Read the model definition and answer for the solid it produces. Units are mm, in the model's axes. A direction names the side the tool comes from. Give positions to 0.01 mm unless a question says otherwise; leave off trailing zeros. Loops run counter-clockwise (first coordinate to the right, second up) from the corner with the lowest first, then second, coordinate; pieces in that order, holes last. Notation, with made-up numbers: (-5.75, -28.75) - (4.25, -28.75) arc R23 ccw to (4.25, -1.75) - close; hole circle Ø5 at (81, -27). An arc over 180 degrees is marked (long way). Use a Markdown table: item, result. Add a question column.
Item 1: A cutting plane is placed at B-B (y = 211.5). Give the number of separate pieces and of enclosed holes in the cut face, plus the area to 3 significant figures.
Item 2: Each of these flat-tipped pins is pushed along its axis until it touches: P1, Ø12, axis at x = 0, y = 342.5, coming from the -Z side; P2, Ø2.5, axis at x = 0, y = 119.5, coming from the +Z side; P3, Ø2.5, axis at x = -0.5, y = 263.5, coming from the -Z side. Where does it stop, or does it pass through?
Item 3: A cutting plane is placed at A-A (x = -0.25). Determine the outline of the cut face in (y, z), plus the area to 3 significant figures.
Item 4: For a pull along X with two mould halves and no side action, classify faces 1 (the face through (-3.5, 203, 0)), 2 (the face through (-5, 203, 0)), 3 (the face through (15, 197, -11)), 4 (the face through (0, 203, 5)) as +X half, -X half, draft (parallel to the pull), parting line (faces both ways), or undercut.
Item 5: Which of the six approach directions +Z, -Z, +X, -X, +Y, -Y give full straight-line access (tool end or side, diameter ignored) to faces 5 (the face through (5, 203, 0)), 6 (the face through (0, 203, 3.5)), 7 (the face through (0, 203, -5)), 8 (the face through (-0.1, 400, -4.5)), 9 (the face through (15, 197, 11))?
Item 6: Consider probe 1 along Z at (x, y) = (11.75, 310.5); probe 2 along X at (y, z) = (219, 1.25); probe 3 along X at (y, z) = (240, 7.5). Determine where each line is inside the solid, lowest interval first. Write a range as [from, to].
from build123d import *

# Parameters (mm, degrees)
SKETCH_1_W          = 30
SKETCH_1_H          = 30
EXTRUDE_1_DEPTH     = 400
CUT_EXTRUDE_1_DEPTH = 400
SKETCH_3_W          = 7
SKETCH_3_H          = 7
SKETCH_3_W_2        = 2.5
SKETCH_3_H_2        = 2.5
CUT_EXTRUDE_2_DEPTH = 400


with BuildPart() as part:
    # 草图1 → 凸台-拉伸1 (new body)
    with BuildSketch(Plane(origin=(0, 0, 0), x_dir=(1, 0, 0), z_dir=(0, 1, 0))):
        Rectangle(SKETCH_1_W, SKETCH_1_H)
    extrude(amount=EXTRUDE_1_DEPTH)

    # 草图2 → 切除-拉伸1 (cut)
    with BuildSketch(Plane(origin=(0, 400, 0), x_dir=(1, 0, 0), z_dir=(0, 1, 0))):
        Polygon((-4.004617846, 5), (4.004617846, 5), (9.97363434, 10.969016494), (9.97363434, 13.177944766), (6.476155555, 13.177944766), (5.84989743, 12.551686641), (5.001284858, 13.400299213), (6.600985645, 15), (-6.600985645, 15), (-5.001284858, 13.400299213), (-5.84989743, 12.551686641), (-6.476155555, 13.177944766), (-9.97363434, 13.177944766), (-9.97363434, 10.969016494), align=None)
        Polygon((10.969016494, 9.97363434), (5, 4.004617846), (5, -4.004617846), (10.969016494, -9.97363434), (13.177944766, -9.97363434), (13.177944766, -6.476155555), (12.551686641, -5.84989743), (13.400299213, -5.001284858), (15, -6.600985645), (15, 6.600985645), (13.400299213, 5.001284858), (12.551686641, 5.84989743), (13.177944766, 6.476155555), (13.177944766, 9.97363434), align=None)
        Polygon((-5, -4.004617846), (-5, 4.004617846), (-10.969016494, 9.97363434), (-13.177944766, 9.97363434), (-13.177944766, 6.476155555), (-12.551686641, 5.84989743), (-13.400299213, 5.001284858), (-15, 6.600985645), (-15, -6.600985645), (-13.400299213, -5.001284858), (-12.551686641, -5.84989743), (-13.177944766, -6.476155555), (-13.177944766, -9.97363434), (-10.969016494, -9.97363434), align=None)
        Polygon((9.97363434, -10.969016494), (4.004617846, -5), (-4.004617846, -5), (-9.97363434, -10.969016494), (-9.97363434, -13.177944766), (-6.476155555, -13.177944766), (-5.84989743, -12.551686641), (-5.001284858, -13.400299213), (-6.600985645, -15), (6.600985645, -15), (5.001284858, -13.400299213), (5.84989743, -12.551686641), (6.476155555, -13.177944766), (9.97363434, -13.177944766), align=None)
    extrude(amount=-CUT_EXTRUDE_1_DEPTH, mode=Mode.SUBTRACT)

    # 草图3 → 切除-拉伸2 (cut)
    with BuildSketch(Plane(origin=(0, 400, 0), x_dir=(1, 0, 0), z_dir=(0, 1, 0))):
        Rectangle(SKETCH_3_W, SKETCH_3_H)
        with Locations((12.48681717, -12.48681717)):
            Rectangle(SKETCH_3_W_2, SKETCH_3_H_2)
        with Locations((12.48681717, 12.48681717)):
            Rectangle(SKETCH_3_W_2, SKETCH_3_H_2)
        with Locations((-12.48681717, -12.48681717)):
            Rectangle(SKETCH_3_W_2, SKETCH_3_H_2)
        with Locations((-12.48681717, 12.48681717)):
            Rectangle(SKETCH_3_W_2, SKETCH_3_H_2)
    extrude(amount=-CUT_EXTRUDE_2_DEPTH, mode=Mode.SUBTRACT)


solid = part.part
Geometry says:
| question | item | result |
|---|---|---|
| 1 | separate pieces | 1 |
| 1 | enclosed holes | 5 |
| 1 | area | 236 mm² |
| 2 | P1 | z = -14.4 |
| 2 | P2 | z = 5 |
| 2 | P3 | z = -5 |
| 3 | outline | (0, -5) - (400, -5) - (400, -3.5) - (0, -3.5) - close; (0, 3.5) - (400, 3.5) - (400, 5) - (0, 5) - close |
| 3 | area | 1,200 mm² |
| 4 | face 1 | undercut |
| 4 | face 2 | -X half |
| 4 | face 3 | +X half |
| 4 | face 4 | undercut |
| 5 | face 5 | +X, +Y, -Y |
| 5 | face 6 | +Y, -Y |
| 5 | face 7 | -Z, +Y, -Y |
| 5 | face 8 | +Z, -Z, +X, -X, +Y |
| 5 | face 9 | +Z, -Z, +X, +Y, -Y |
| 6 | probe 1 | [-15, -13.74], [-11.24, -9.97], [9.97, 11.24], [13.74, 15] |
| 6 | probe 2 | [-5, -3.5], [3.5, 5] |
| 6 | probe 3 | [-15, -13.18], [-8.5, -6.5], [6.5, 8.5], [13.18, 15] |
